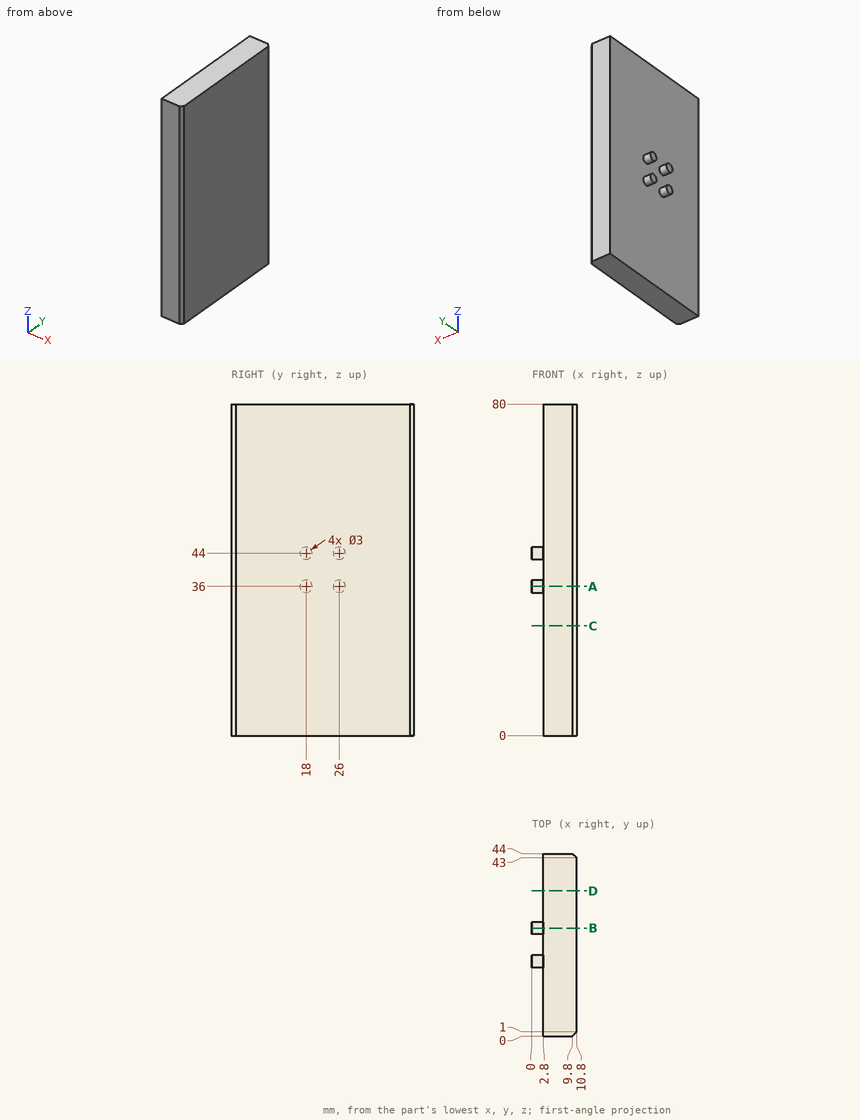
The figure shows three views and two pictorial views of one solid part (mm, origin at its lowest corner). Answer the questions. Coordinates: 2 decimals unless noted, no trailing zeros. Loops run counter-clockwise (first coordinate to the right, second up) from the corner with the lowest first, then second, coordinate; pieces in that order, holes last. Notation, with made-up numbers: M 89.25,9 L 113.25,9 A22 cw 113.25,48 Z; hole C 52.5,72.5 d5. An arc over 180 degrees is marked long. Answer as CSV lines item,"result". Start each with the question number.
(1) The part is cut by section A-A (z = 36). Give the vertices of the cut face in (x, y), and give its area (3 significant figures).
(2) Given pin 1 (13 mm diameter, centred on y = 17, z = 52, fed in from -X); pin 2 (1.5 mm diameter, centred on x = 8, y = 6.5, fed in from -Z), each flat-ended and moving along its own axis, determine where each tip first touches the part or whether it passes through.
(3) The part is cut by section D-D (y = 35). Give the vertices of the cut face in (x, z).
(4) The part is cut by section B-B (y = 26). Give the vertices of the cut face in (x, z), and give its area (3 significant figures).
(5) The part is cut by section C-C (z = 26.5). Give the vertices of the cut face in (x, y), and give its area (3 significant figures).
(6) Find the intervals of material crossed by L1, parallel to X at y = 28.5, z = 30.5; L2, parallel to Z at x = 0.75, y = 27; L3, parallel to Y at x = 10, z = 35, in increasing order. Write a range as [from, to].
Determined:
1,outline,"M 0,16.5 L 2.8,16.5 L 2.8,0 L 9.8,0 L 10.8,1 L 10.8,43 L 9.8,44 L 2.8,44 L 2.8,27.5 L 0,27.5 L 0,24.5 L 2.8,24.5 L 2.8,19.5 L 0,19.5 Z"
1,area,"368 mm2"
2,pin 1,"x = 2.8"
2,pin 2,"z = 0"
3,outline,"M 2.8,0 L 10.8,0 L 10.8,80 L 2.8,80 Z"
4,outline,"M 0,34.5 L 2.8,34.5 L 2.8,0 L 10.8,0 L 10.8,80 L 2.8,80 L 2.8,45.5 L 0,45.5 L 0,42.5 L 2.8,42.5 L 2.8,37.5 L 0,37.5 Z"
4,area,"657 mm2"
5,outline,"M 2.8,0 L 9.8,0 L 10.8,1 L 10.8,43 L 9.8,44 L 2.8,44 Z"
5,area,"351 mm2"
6,L1,"[2.8, 10.8]"
6,L2,"[34.88, 37.12], [42.88, 45.12]"
6,L3,"[0.2, 43.8]"
